Design review of the part shown in the three views and the two pictorial views. Dimensions are in mm from the part's minimum x, y and z. A direction names the side the tool comes from. Give positions to 0.01 mm unless a question says otherwise; leave off trailing zeros. Order: outer loops, then holes, each group sorted by start corner. A loop starts at its lowest first (then second) coordinate and runs counter-clockwise, first axis right, second up.
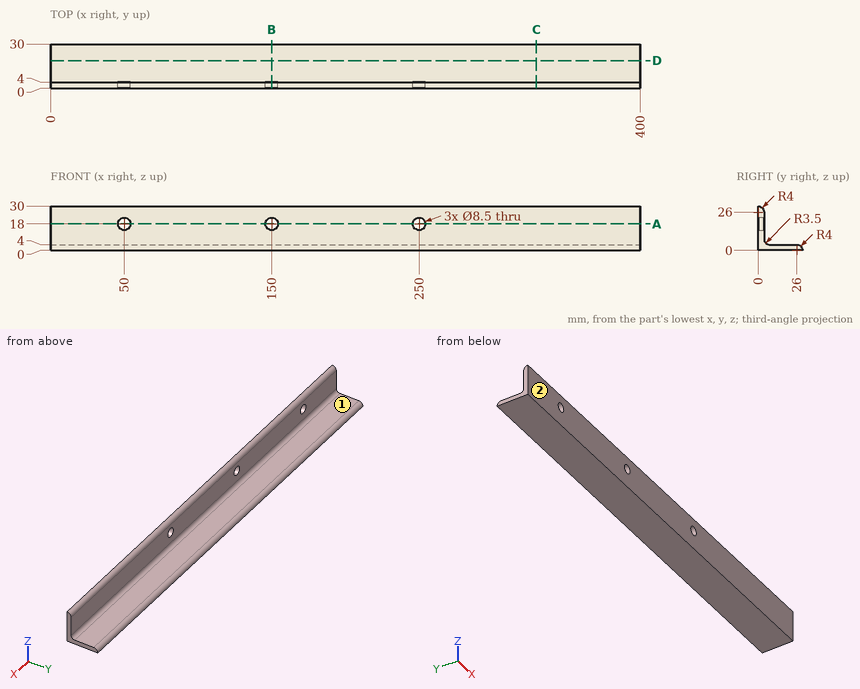
Item 1: Take a section at C-C (x = 329.5). Give the boundary of the cut face in (y, z), and give its area (3 significant figures).
Values found:
outline: (0, 0) - (30, 0) arc R4 ccw to (26, 4) - (7.5, 4) arc R3.5 cw to (4, 7.5) - (4, 26) arc R4 ccw to (0, 30) - close
area: 220 mm2
Item 2: Take a section at A-A (z = 18). Give the boundary of the cut face in (x, y), and give its area (3 significant figures).
Values found:
outline: (0, 0) - (45.75, 0) - (45.75, 4) - (0, 4) - close; (54.25, 0) - (145.75, 0) - (145.75, 4) - (54.25, 4) - close; (154.25, 0) - (245.75, 0) - (245.75, 4) - (154.25, 4) - close; (254.25, 0) - (400, 0) - (400, 4) - (254.25, 4) - close
area: 1,500 mm2
Item 3: Take a section at B-B (x = 150). Give the boundary of the cut face in (y, z), and give its area (3 significant figures).
Values found:
outline: (0, 0) - (30, 0) arc R4 ccw to (26, 4) - (7.5, 4) arc R3.5 cw to (4, 7.5) - (4, 13.75) - (0, 13.75) - close; (0, 22.25) - (4, 22.25) - (4, 26) arc R4 ccw to (0, 30) - close
area: 186 mm2
Item 4: Clearance check with flat-ended pins moving along their axes: pin 1 Ø1.5 at (x, y) = (332.5, 8) entering from +Z; pin 2 Ø5 at (x, z) = (50, 18) entering from +Y; pin 3 Ø1 at (x, z) = (299.5, 14) entering from +Y; pin 4 Ø2 at (x, z) = (169.5, 3.5) entering from +Y. State where each tip first meets the part, or that it passes through.
Values found:
pin 1: stops at z = 4.01
pin 2: passes through
pin 3: stops at y = 4
pin 4: stops at y = 29.12
Item 5: For the marked faces 1 and 2, list the 3-axis set-ups (+Z, -Z, +X, -X, +Y, -Y) from which the entire face can be reached by the end or side of a thin tool; tool diameter is ignored.
Values found:
face 1: +Z, +X, -X, +Y
face 2: +Z, -Z, +X, -X, -Y
Item 6: For line 1 (X direction, y = 1.9, z = 18); line 2 (Z direction, x = 122.5, y = 25); line 3 (Y direction, x = 275.5, z = 26.5), list the stretches that pass through material, from the lowest coordinate up.
Values found:
line 1: x = 0 to 45.75, 54.25 to 145.75, 154.25 to 245.75, 254.25 to 400
line 2: z = 0 to 4
line 3: y = 0 to 3.97
Item 7: Take a section at D-D (y = 18.75). Give the boundary of the cut face in (x, z), and give its area (3 significant figures).
Values found:
outline: (0, 0) - (400, 0) - (400, 4) - (0, 4) - close
area: 1,600 mm2
